```python
from build123d import *

# Parameters (mm, degrees)
F1_DEPTH  = 102
F2_R      = 50.99999
F3_R      = 27
F3_R_2    = 18.5
F4_DEPTH  = 30
F5_R      = 18.5
F6_DEPTH  = 30
F7_R      = 10
F8_DEPTH  = 30
F11_DEPTH = 12.5
F12_R     = 20


# Not quite as in the source:
# - a fillet or chamfer is up to 0.001 mm smaller than in the source, because OpenCascade refuses the exact size


with BuildPart() as f1:
    # F0 (on Front) → F1 (new body)
    with BuildSketch(Plane.XZ):
        Polygon((-36.2992759747, -102.7012261555), (-145.2992759747, -102.7012261555), (-145.2992759747, -128.7012261555), (-21.2881689757, -128.7012261555), (94.2118310243, 71.3506421187), (71.6951705259, 84.3506421187), align=None)
    extrude(amount=F1_DEPTH)

    # F2 (radius 51 in the source; OpenCascade refuses exactly that, so slightly less here)
    f2_edges = [f1.edges().sort_by_distance(p)[0] for p in [
        (82.953501, 0, 77.850642),
        (82.953501, -102, 77.850642),
    ]]
    fillet(f2_edges, radius=F2_R)

    # F3 (on face) → F4 (join)
    with BuildSketch(Plane(origin=(17.2464784442, 0, -9.9572589724), x_dir=(0, -1, 0), z_dir=(-0.8660254038, 0, 0.5))):
        with Locations((51, 57.8973841632)):
            Circle(F3_R)
        with Locations((51, 57.8973841632)):
            Circle(F3_R_2, mode=Mode.SUBTRACT)
    extrude(amount=F4_DEPTH)

    # F5 (on face) → F6 (cut)
    with BuildSketch(Plane(origin=(17.2464784442, 0, -9.9572589724), x_dir=(0, -1, 0), z_dir=(-0.8660254038, 0, 0.5))):
        with Locations((51, 57.8973841632)):
            Circle(F5_R)
    extrude(amount=-F6_DEPTH, mode=Mode.SUBTRACT)

    # F7 (on face) → F8 (cut)
    with BuildSketch(Plane.XY.offset(-102.7012261555)):
        with Locations((-125.2992759747, -20)):
            Circle(F7_R)
        with Locations((-125.2992759747, -82)):
            Circle(F7_R)
        with Locations((-56.2992759747, -20)):
            Circle(F7_R)
        with Locations((-56.2992759747, -82)):
            Circle(F7_R)
    extrude(amount=-F8_DEPTH, mode=Mode.SUBTRACT)

    # F10 (on offset) → F11 (join, symmetric)
    with BuildSketch(Plane.XZ.offset(51)):
        Polygon((-35.6261391794, -102.7012261555), (1.8678903299, -36.5937549351), (-145.2992759747, -102.7012261555), align=None)
    extrude(amount=F11_DEPTH, both=True)

    # F12
    f12_edges = [f1.edges().sort_by_distance(p)[0] for p in [
        (-145.299276, 0, -115.701226),
        (-145.299276, -102, -115.701226),
    ]]
    fillet(f12_edges, radius=F12_R)


solid = f1.part
```
CAD build for the part. Positions are in the model's coordinates, mm. A direction names the side the tool comes from. Give positions to 0.01 mm unless a question says otherwise; leave off trailing zeros. Loops run counter-clockwise (first coordinate to the right, second up) from the corner with the lowest first, then second, coordinate; pieces in that order, holes last. Notation, with made-up numbers: (50, 76.25) - (95, 76.25) arc R11 cw to (95, 90.25) - close; hole circle Ø8 at (-26.5, 84.25). An arc over 180 degrees is marked (long way). Put each result on its own line as item: value.
Q1. Slice it at A-A (x = -58.5). Give the cut face in (y, z).
Filled in:
outline: (-102, -128.7) - (-91.75, -128.7) - (-91.75, -102.7) - (-102, -102.7) - close; (-72.25, -128.7) - (-29.75, -128.7) - (-29.75, -102.7) - (-38.5, -102.7) - (-38.5, -63.71) - (-63.5, -63.71) - (-63.5, -102.7) - (-72.25, -102.7) - close; (-10.25, -128.7) - (0, -128.7) - (0, -102.7) - (-10.25, -102.7) - close
Q2. Flat gauge pins, fed straight in: pin 1 (12 mm diameter, centred on y = -53, z = 38, fed in from +X); pin 2 (11.5 mm diameter, centred on x = -99, y = -87.5, fed in from +Z); pin 3 (1.5 mm diameter, centred on y = -24, z = 6, fed in from -X); pin 4 (12 mm diameter, centred on x = -56.3, y = -82, fed in from -Z). Where does each tip first touch, or does it go through?
Filled in:
pin 1: stops at x = 78.42
pin 2: stops at z = -102.7
pin 3: stops at x = 26.03
pin 4: passes through
Q3. Slice it at B-B (y = -16). Give the cut face in (x, z), plus the area to 3 significant figures.
Filled in:
outline: (-144.9, -128.7) - (-134.46, -128.7) - (-134.46, -102.7) - (-144.9, -102.7) - close; (-116.13, -128.7) - (-65.46, -128.7) - (-65.46, -102.7) - (-116.13, -102.7) - close; (-47.13, -128.7) - (-21.29, -128.7) - (87.26, 59.31) - (64.74, 72.31) - (-36.3, -102.7) - (-47.13, -102.7) - close
area: 7,510 mm²
Q4. Slice it at C-C (z = -62.5). Give the cut face in (x, y), plus the area to 3 significant figures.
Filled in:
outline: (-55.8, -63.5) - (-13.09, -63.5) - (-13.09, -102) - (16.93, -102) - (16.93, 0) - (-13.09, 0) - (-13.09, -38.5) - (-55.8, -38.5) - close
area: 4,130 mm²
Q5. Probe line 1 along Z through (x, y) = (31, -42); line 2 along Y through (x, z) = (-81, -78.5); line 3 along Y through (x, z) = (56.5, 51). List the from-to ranges inside material, lowest first.
Filled in:
line 1: z = -38.14 to 13.86, 19.56 to 30.29, 67.62 to 73.86
line 2: y = -63.5 to -38.5
line 3: y = -99.89 to -62.46, -39.54 to -2.11
Q6. Mould opens along Y. For faces 4 (the face through (-61, -63.5, -82)), 5 (the face through (-145.299, -51, -116)), 6 (the face through (-63.67, -75.24, -115.52)), 7 (the face through (75.524, -15.336, 65.347)) say: pulls with the +Y half, pulls with the -Y half, needs draft (parallel to the pull), parting line crosses it, or undercut.
Filled in:
face 4: pulls with the -Y half
face 5: needs draft
face 6: undercut
face 7: pulls with the +Y half
Q7. Tool access for faces 1 (the face through (-90, -82, -102.701)), 2 (the face through (-70.686, -51.175, -69.185)), 3 (the face through (-61, -38.5, -82)): list every direction of +Z, -Z, +X, -X, +Y, -Y with a clear straight run to the whole face (end or side of a thin tool).
Filled in:
face 1: +Z, -X, -Y
face 2: +Z, -X, +Y, -Y
face 3: +Z, -X, +Y
